The model under review builds one solid part; all positions refer to its coordinate system, in mm. Round coordinates to 2 decimals unless told otherwise and drop trailing zeros. Order: outer loops, then holes, each group sorted by start corner. A loop starts at its lowest first (then second) coordinate and runs counter-clockwise, first axis right, second up.
1) Clearance check with flat-ended pins moving along their axes: P1, Ø5, axis at x = 63, z = 23.5, coming from the -Y side; P2, Ø2, axis at y = 0.5, z = 23.5, coming from the +X side. State where each tip first meets the part, or that it passes through.
2) Consider section A-A (x = -17.5). Give the boundary of the cut face in (y, z), then the cut area to 3 significant figures.
3) Consider section B-B (y = 1.05). Give the boundary of the cut face in (x, z), then the cut area to 3 significant figures.
4) Consider section C-C (z = 54.5). Give the boundary of the cut face in (x, y).
5) Consider section D-D (z = -26). Give the boundary of the cut face in (x, y), then the cut area to 3 significant figures.
6) To check wall thickness, follow L1, parallel to Z at x = -39, y = 2.15; L2, parallel to Z at x = 62.5, y = 1.4; L3, parallel to X at y = 2.35, z = -48. State the ranges of each line that lie inside material, in increasing order.
from build123d import *

# Parameters (mm, degrees)
ESQUISSE1_W              = 148
ESQUISSE1_H              = 148
BOSS_EXTRU_1_DEPTH       = 4
CONG_1_R                 = 2
ESQUISSE12_W             = 23.640980831
ESQUISSE12_H             = 10
ESQUISSE12_W_2           = 17.131931469
ENL_V_MAT_EXTRU_12_DEPTH = 2
ESQUISSE13_W             = 38.5
ESQUISSE13_H             = 18.5
ENL_V_MAT_EXTRU_13_DEPTH = 5


with BuildPart() as part:
    # Esquisse1 → Boss.-Extru.1 (new body)
    with BuildSketch(Plane(origin=(0, 0, 0), x_dir=(1, 0, 0), z_dir=(0, 1, 0))):
        Rectangle(ESQUISSE1_W, ESQUISSE1_H)
    extrude(amount=BOSS_EXTRU_1_DEPTH)

    # Congé1
    cong_1_edges = [part.edges().sort_by_distance(p)[0] for p in [
        (-74, 2, 74),
        (-74, 2, -74),
    ]]
    fillet(cong_1_edges, radius=CONG_1_R)

    # Esquisse12 → Enlèv. mat.-Extru.12 (cut)
    with BuildSketch(Plane(origin=(0, 0, 0), x_dir=(1, 0, 0), z_dir=(0, 1, 0))):
        with Locations((68.740682109, -25.384218458)):
            Rectangle(ESQUISSE12_W, ESQUISSE12_H)
        with Locations((65.486157429, 24.615781542)):
            Rectangle(ESQUISSE12_W_2, ESQUISSE12_H)
    extrude(amount=ENL_V_MAT_EXTRU_12_DEPTH, mode=Mode.SUBTRACT)

    # Esquisse13 → Enlèv. mat.-Extru.13 (cut)
    with BuildSketch(Plane(origin=(0, 0, 0), x_dir=(1, 0, 0), z_dir=(0, 1, 0))):
        with Locations((-34.75, -54.75)):
            Rectangle(ESQUISSE13_W, ESQUISSE13_H)
        with Locations((-34.75, 54.75)):
            Rectangle(ESQUISSE13_W, ESQUISSE13_H)
    extrude(amount=ENL_V_MAT_EXTRU_13_DEPTH, mode=Mode.SUBTRACT)


solid = part.part
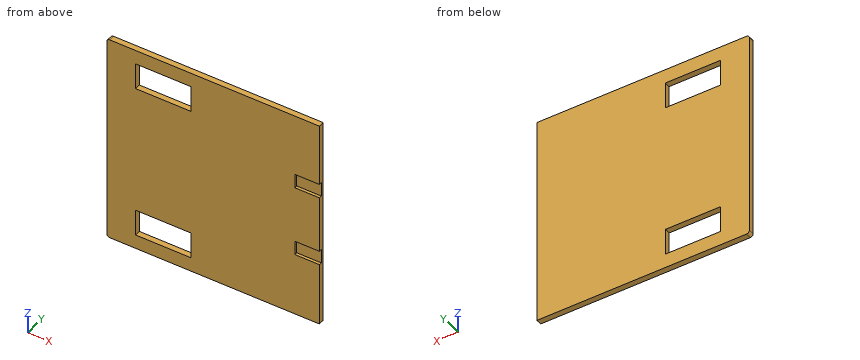
Answer below:
1. P1: stops at y = 2
1. P2: stops at x = 56.92
2. outline: (0, -74) - (4, -74) - (4, -64) - (0, -64) - close; (0, -45.5) - (4, -45.5) - (4, 45.5) - (0, 45.5) - close; (0, 64) - (4, 64) - (4, 74) - (0, 74) - close
2. area: 444 mm2
3. outline: (-74, -72) arc R2 ccw to (-72, -74) - (74, -74) - (74, -29.62) - (56.92, -29.62) - (56.92, -19.62) - (74, -19.62) - (74, 20.38) - (56.92, 20.38) - (56.92, 30.38) - (74, 30.38) - (74, 74) - (-72, 74) arc R2 ccw to (-74, 72) - close; hole (-54, -64) - (-15.5, -64) - (-15.5, -45.5) - (-54, -45.5) - close; hole (-54, 45.5) - (-15.5, 45.5) - (-15.5, 64) - (-54, 64) - close
3. area: 20,100 mm2
4. outline: (-74, 0) - (-54, 0) - (-54, 4) - (-74, 4) - close; (-15.5, 0) - (74, 0) - (74, 4) - (-15.5, 4) - close
5. outline: (-74, 0) - (56.92, 0) - (56.92, 2) - (74, 2) - (74, 4) - (-74, 4) - close
5. area: 558 mm2
6. L1: z = -74 to -64, -45.5 to 45.5, 64 to 74
6. L2: z = -74 to -29.62, -19.62 to 20.38, 30.38 to 74
6. L3: x = -74 to -54, -15.5 to 74
